Design review of the part built by this model. Coordinates are the model's own, in mm. A direction names the side the tool comes from. Coordinates: 2 decimals unless noted, no trailing zeros. Write each loop counter-clockwise with the first axis right and the second up, starting at its lowest first coordinate (ties: lowest second). Pieces come first, ordered by that corner, then holes. Notation, with made-up numbers: (-14.5, 61.5) -> (11.5, 61.5) arc R15 ccw to (11.5, 77.5) -> close; hole circle Ø11 at (-39.5, 89.5). An arc over 180 degrees is marked (long way). Answer in a Markdown table with one row per item. Add a question column.
Item 1: Take a section at C-C, the plane z = -16.5. Write out the cut boundary in (x, y).
Item 2: To check wall thickness, follow line 1 (Z direction, x = 4, y = 1.5); line 2 (Z direction, x = -4.5, y = 6.5); line 3 (Y direction, x = -0.25, z = -13). State the ranges of each line that lie inside material, in increasing order.
Item 3: Take a section at A-A, the plane y = 0. Write out the cut boundary in (x, z), and give its area (3 significant figures).
Item 4: Take a section at D-D, the plane z = -6. Write out the cut boundary in (x, y).
Item 5: Clearance check with flat-ended pins moving along their axes: P1, Ø5.5, axis at y = 0, z = -30, coming from the +X side; P2, Ø8, axis at x = 5, z = -20.5, coming from the +Y side; P3, Ø5, axis at y = -1.5, z = -18.5, coming from the -X side. State where each tip first meets the part, or that it passes through.
Item 6: For faces 4 (the face through (-2, 7, 0)), 5 (the face through (0, 2.935, -28)), 6 (the face through (-0.681, 0, -27.8)), list the 3-axis set-ups (+Z, -Z, +X, -X, +Y, -Y) from which the entire face can be reached by the end or side of a thin tool; tool diameter is ignored.
Item 7: Draft analysis for pull direction Y (two halves, no side actions). For faces 1 (the face through (3.746, 0.165, -19.395)), 2 (the face through (0, 0, 12)), 3 (the face through (0.121, 0.065, -27.985)), state which applies: released by +Y, released by -Y, zero draft, split by the parting line, or undercut.
Item 8: Take a section at B-B, the plane x = 0. Write out the cut boundary in (y, z).
from build123d import *

# Parameters (mm, degrees)
SKETCH_1_R          = 8.5
EXTRUDE_1_DEPTH     = 5
SKETCH_2_R          = 7
EXTRUDE_2_DEPTH     = 7
EXTRUDE_2_TAPER     = 5
SKETCH_3_R          = 7
EXTRUDE_3_DEPTH     = 12
SKETCH_4_R          = 3.75
EXTRUDE_4_DEPTH     = 15
SKETCH_5_W          = 1.582755529
SKETCH_5_H          = 5.869385088
EXTRUDE_5_DEPTH     = 5
SKETCH_6_R          = 1.484108277
CUT_EXTRUDE_1_DEPTH = 5
FILLET_1_R          = 2
SKETCH_7_R          = 0.75
EXTRUDE_6_DEPTH     = 1.5


with BuildPart() as part:
    # Эскиз1 → Бобышка-Вытянуть1 (new body)
    with BuildSketch(Plane.XY):
        Circle(SKETCH_1_R)
    extrude(amount=EXTRUDE_1_DEPTH)

    # Эскиз2 → Бобышка-Вытянуть2 (add)
    with BuildSketch(Plane.XY.offset(5)):
        Circle(SKETCH_2_R)
    extrude(amount=EXTRUDE_2_DEPTH, taper=EXTRUDE_2_TAPER)

    # Эскиз3 → Бобышка-Вытянуть3 (add)
    with BuildSketch(Plane(origin=(0, 0, 0), x_dir=(-1, 0, 0), z_dir=(0, 0, -1))):
        with Locations(Location((0, 0, 0), (0, 0, 180))):
            Circle(SKETCH_3_R)
    extrude(amount=EXTRUDE_3_DEPTH)

    # Эскиз4 → Бобышка-Вытянуть4 (add)
    with BuildSketch(Plane(origin=(0, 0, -12), x_dir=(-1, 0, 0), z_dir=(0, 0, -1))):
        Circle(SKETCH_4_R)
    extrude(amount=EXTRUDE_4_DEPTH)

    # Эскиз5 → Бобышка-Вытянуть5 (add)
    with BuildSketch(Plane(origin=(0, 0, -27), x_dir=(-1, 0, 0), z_dir=(0, 0, -1))):
        with Locations((-0.109913578, 0)):
            Rectangle(SKETCH_5_W, SKETCH_5_H)
    extrude(amount=EXTRUDE_5_DEPTH)

    # Эскиз6 → Вырез-Вытянуть1 (cut)
    with BuildSketch(Plane(origin=(0.901291343, 0, 0), x_dir=(0, 0, -1), z_dir=(1, 0, 0))):
        with Locations((29.467495163, 0)):
            Circle(SKETCH_6_R)
    extrude(amount=-CUT_EXTRUDE_1_DEPTH, mode=Mode.SUBTRACT)

    # Скругление1
    fillet_1_edges = [part.edges().sort_by_distance(p)[0] for p in [
        (0.109913578, -2.934692544, -32),
        (0.109913578, 2.934692544, -32),
    ]]
    fillet(fillet_1_edges, radius=FILLET_1_R)

    # Эскиз7 → Бобышка-Вытянуть6 (add)
    with BuildSketch(Plane(origin=(0, 0, 0), x_dir=(-1, 0, 0), z_dir=(0, 0, -1))):
        with Locations((0, 7.010668314)):
            Circle(SKETCH_7_R)
    extrude(amount=EXTRUDE_6_DEPTH)


solid = part.part
Answers:
| question | item | result |
|---|---|---|
| 1 | outline | circle Ø7.5 at (0, 0) |
| 2 | line 1 | z = -12 to 12 |
| 2 | line 2 | z = 0 to 5 |
| 2 | line 3 | y = -3.74 to 3.74 |
| 3 | outline | (-8.5, 0) -> (-7, 0) -> (-7, -12) -> (-3.75, -12) -> (-3.75, -27) -> (-0.68, -27) -> (-0.68, -27.98) -> (0.9, -27.98) -> (0.9, -27) -> (3.75, -27) -> (3.75, -12) -> (7, -12) -> (7, 0) -> (8.5, 0) -> (8.5, 5) -> (7, 5) -> (6.39, 12) -> (-6.39, 12) -> (-7, 5) -> (-8.5, 5) -> close; (-0.68, -32) -> (0.9, -32) -> (0.9, -30.95) -> (-0.68, -30.95) -> close |
| 3 | area | 462 mm^2 |
| 4 | outline | circle Ø14 at (0, 0) |
| 5 | P1 | stops at x = 0.9 |
| 5 | P2 | stops at y = 3.61 |
| 5 | P3 | stops at x = -3.75 |
| 6 | face 4 | -Z |
| 6 | face 5 | -Z, +X, -X, +Y |
| 6 | face 6 | -Z, -X, +Y, -Y |
| 7 | face 1 | split by the parting line |
| 7 | face 2 | zero draft |
| 7 | face 3 | undercut |
| 8 | outline | (-8.5, 0) -> (-7, 0) -> (-7, -12) -> (-3.75, -12) -> (-3.75, -27) -> (-2.93, -27) -> (-2.93, -30) arc R2 ccw to (-0.93, -32) -> (0.93, -32) arc R2 ccw to (2.93, -30) -> (2.93, -27) -> (3.75, -27) -> (3.75, -12) -> (7, -12) -> (7, -1.5) -> (7.76, -1.5) -> (7.76, 0) -> (8.5, 0) -> (8.5, 5) -> (7, 5) -> (6.39, 12) -> (-6.39, 12) -> (-7, 5) -> (-8.5, 5) -> close; hole circle Ø2.97 at (0, -29.47) |
